from build123d import *

# Parameters (mm, degrees)
F0_W     = 92.075
F0_H     = 92.075
F0_R     = 38.1
F1_DEPTH = 152.4
F2_DEPTH = 19.05
F3_R     = 1.5875


with BuildPart() as f1:
    # F0 (on Front) → F1 (new body)
    with BuildSketch(Plane.XZ):
        Rectangle(F0_W, F0_H)
        Circle(F0_R, mode=Mode.SUBTRACT)
    extrude(amount=-F1_DEPTH)

    # F0 (on Front) → F2 (join)
    with BuildSketch(Plane.XZ):
        Rectangle(F0_W, F0_H)
        Circle(F0_R, mode=Mode.SUBTRACT)
        Circle(F0_R)
    extrude(amount=-F2_DEPTH)

    # F3
    f3_edges = [f1.edges().sort_by_distance(p)[0] for p in [
        (-46.0375, 76.2, 46.0375),
        (-46.0375, 76.2, -46.0375),
        (46.0375, 76.2, 46.0375),
        (46.0375, 0, 0),
        (46.0375, 76.2, -46.0375),
        (46.0375, 152.4, 0),
        (0, 0, 46.0375),
        (-46.0375, 0, 0),
        (0, 0, -46.0375),
        (0, 152.4, -46.0375),
        (-46.0375, 152.4, 0),
        (0, 152.4, 46.0375),
        (-38.1, 152.4, 0),
    ]]
    fillet(f3_edges, radius=F3_R)


solid = f1.part
Design review of the part built by this model. Coordinates are the model's own, in mm. A direction names the side the tool comes from. Round coordinates to 2 decimals unless told otherwise and drop trailing zeros. One line per item, written item: value. Start each with the question number.
Q1. Tool access review of faces 4 (the face through (-30.235, 84.009, -23.183)), 5 (the face through (-1, 152.4, 40)): name each direction out of +Z, -Z, +X, -X, +Y, -Y from which nothing blocks a thin tool from reaching the whole face with its end or side.
Q2. Insertion check: P1, Ø3, axis at x = -13.5, z = 22.5, coming from the +Y side. The pin has a flat end and moves straight along its axis. Give the tip position at first contact, or say it passes through.
Q3. To check wall thickness, follow probe 1 along X at (y, z) = (40, -1); probe 2 along Z at (x, y) = (0, 66.5); probe 3 along Y at (x, z) = (0, 10.5). State the ranges of each line that lie inside material, in increasing order.
Q4. The part is to be moulded in two halves that separate along X. For faces 1 (the face through (46.038, 75, -1)), 2 (the face through (-1, 75, -46.038)), 3 (the face through (-1, 19.05, 1)), say which applies: pulls with the +X half, pulls with the -X half, needs draft (parallel to the pull), parting line crosses it, or undercut.
Response:
1. face 4: +Y
1. face 5: +Z, -Z, +X, -X, +Y
2. P1: stops at y = 19.05
3. probe 1: x = -46.04 to -38.09, 38.09 to 46.04
3. probe 2: z = -46.04 to -38.1, 38.1 to 46.04
3. probe 3: y = 0 to 19.05
4. face 1: pulls with the +X half
4. face 2: needs draft
4. face 3: undercut
